Autodesk Inventor part; units mm, degrees
ref_plane "YZ Plane" through (0, 0, 0) normal (1, 0, 0) x (0, 1, 0)
ref_plane "XZ Plane" through (0, 0, 0) normal (0, 1, 0) x (-1, 0, 0)
ref_plane "XY Plane" through (0, 0, 0) normal (0, 0, 1) x (1, 0, 0)
sketch "Sketch1" plane through (0, 0, 0) normal (0, 1, 0) x (-1, 0, 0)
  line L0 (5, 5) -> (-5, 5)
  line L1 (-5, 5) -> (-5, -5)
  line L2 (-5, -5) -> (5, -5)
  line L3 (5, -5) -> (5, 5)
  line L4 (6, 6) -> (-6, 6)
  line L5 (-6, 6) -> (-6, -6)
  line L6 (-6, -6) -> (6, -6)
  line L7 (6, -6) -> (6, 6)
  point P0 (0, 0)
  dimension "d0" = 10
  dimension "d1" = 10
  dimension "d2" = 5
  dimension "d3" = 5
  dimension "d4" = 12
  dimension "d5" = 12
  dimension "d6" = 1
  dimension "d7" = 1
extrude "Extrusion1" add sketch "Sketch1" along normal blind 2
sketch "Sketch2" plane through (6, 0, 6) normal (1, 0, 0) x (0, 0, -1)
  line L0 (0, 0) -> (0, 2)
  line L1 (12, 0) -> (12, 2)
  line L2 (0, 2) -> (12, 2)
  line L3 (12, 2) -> (12, 1)
  line L4 (12, 1) -> (0, 1)
  line L5 (0, 1) -> (0, 2)
  point P0 (6, 0)
extrude "Extrusion2" add sketch "Sketch2" against normal blind 11.5
sketch "Sketch3" plane through (0, 2, 0) normal (0, 1, 0) x (1, 0, 0)
  line L0 (-2, -2) -> (2, -2)
  line L1 (2, -2) -> (2, 2)
  line L2 (2, 2) -> (-2, 2)
  line L3 (-2, 2) -> (-2, -2)
  circle A0 centre (0, 0) radius 2.8284
  line L4 (0, -2.8284) -> (-2.8284, 0)
  line L5 (-2.8284, 0) -> (0, 2.8284)
  line L6 (2.8284, 0) -> (0, 2.8284)
  line L7 (2.8284, 0) -> (0, -2.8284)
  point P0 (0.8284, -2)
  point P1 (2, -0.8284)
  point P2 (2, 0.8284)
  point P3 (0.8284, 2)
  point P4 (-0.8284, 2)
  point P5 (-2, 0.8284)
  point P6 (-2, -0.8284)
  point P7 (-0.8284, -2)
  dimension "d13" = 4
  dimension "d14" = 4
  dimension "d15" = 2
  dimension "d16" = 2
extrude "Extrusion3" cut sketch "Sketch3" along normal blind 23.25 and the other way blind 11.625 contours L4 L3 L5 L2 L6 L1 L7 L0
sketch "Sketch4" plane through (0, 2, 0) normal (0, 1, 0) x (1, 0, 0)
  line L0 (2, -0.8284) -> (2, 0.8284)
  line L1 (2, -0.8284) -> (2.8765, -0.8284)
  line L2 (2.8765, -0.8284) -> (2.8765, 0.8284)
  line L3 (2.8765, 0.8284) -> (2, 0.8284)
  line L4 (2, 0.8284) -> (2, -0.8284)
  line L5 (2.8765, -0.8284) -> (7.5124, -0.8284)
  line L6 (7.5124, -0.8284) -> (7.5124, 0.8284)
  line L7 (7.5124, 0.8284) -> (2.8765, 0.8284)
  line L8 (2.8765, 0.8284) -> (2.8765, -0.8284)
  point P0 (0, 0)
  point P1 (2.8765, 0.8284)
  point P2 (2, 0.8284)
extrude "Extrusion4" cut sketch "Sketch4" against normal blind 1
sketch "Sketch5" plane through (0, 2, 0) normal (0, 1, 0) x (1, 0, 0)
  line L0 (-6, -6) -> (6, -6)
  line L1 (6, 0.8284) -> (6, 6)
  line L2 (-6, -6) -> (6, -6)
  line L3 (6, -6) -> (6, 6)
  line L4 (6, 6) -> (-6, 6)
  line L5 (-6, 6) -> (-6, -6)
  point P0 (0, 0)
  point P1 (6, -6)
extrude "Extrusion5" add sketch "Sketch5" along normal blind 25
sketch "Sketch6" plane through (6, 0, 6) normal (1, 0, 0) x (0, 0, -1)
  line L0 (5.1716, 1) -> (5.1716, 2)
  line L1 (5.1716, 2) -> (-3.596, 2)
  line L2 (0, 0) -> (0, 27)
  line L3 (4, 2) -> (5.1716, 2)
  line L4 (5.1716, 2) -> (16.1787, 2)
  line L5 (5.1716, 2) -> (6.8284, 2)
  line L6 (6, 2) -> (6, 6)
  line L7 (0, 2) -> (6, 4)
  line L8 (6, 4) -> (12, 2)
  line L9 (12, 0) -> (12, 27)
  line L10 (12, 2) -> (-2.4689, 2)
  line L11 (-2.4689, 2) -> (-2.4689, 28.669)
  line L12 (-2.4689, 28.669) -> (12, 28.669)
  line L13 (12, 28.669) -> (12, 2)
  point P0 (6, 0)
  dimension "d23" = 4
extrude "Extrusion6" cut sketch "Sketch6" against normal blind 23.25 contours L1 L11 L12 L13 L9 L8 L7
sketch "Sketch7" plane through (-6, 0, 6) normal (0, 0, 1) x (1, 0, 0)
  line L0 (6, 0) -> (6, 4)
  line L1 (12, 4) -> (0, 4)
  line L2 (0, 2) -> (12, 2)
  line L3 (12, 2) -> (6, 4)
  line L4 (0, 4) -> (0, 2)
  line L5 (6, 4) -> (0, 2)
  line L6 (0, 2) -> (13.6732, 2)
  line L7 (13.6732, 2) -> (13.6732, 4.9606)
  line L8 (13.6732, 4.9606) -> (0, 4.9606)
  line L9 (0, 4.9606) -> (0, 2)
extrude "Extrusion7" cut sketch "Sketch7" against normal blind 41.75 contours L5 L4 L1 | L1 L9 L8 L7 L6 L3
sketch "Sketch8" plane through (0, 2, 0) normal (0, -1, 0) x (1, 0, 0)
  line L0 (6, 6) -> (0, 0)
  line L1 (1.9974, 1.9974) -> (-2.0026, 1.9974)
  line L2 (-2.0026, 1.9974) -> (-2.0026, -2.0026)
  line L3 (-2.0026, -2.0026) -> (1.9974, -2.0026)
  line L4 (1.9974, -2.0026) -> (1.9974, 1.9974)
  dimension "d30" = 4
  dimension "d31" = 4
extrude "Extrusion8" cut sketch "Sketch8" against normal blind 105
sketch "Sketch9" plane through (6, 0, 6) normal (1, 0, 0) x (0, 0, -1)
  line L0 (0, 0) -> (0, 2)
  line L1 (12, 0) -> (12, 2)
  line L2 (0, 0) -> (12, 0)
  line L3 (12, 0) -> (12, 2)
  line L4 (12, 2) -> (0, 2)
  line L5 (0, 2) -> (0, 0)
  point P0 (6, 0)
extrude "Extrusion9" add sketch "Sketch9" along normal blind 10
sketch "Sketch10" plane through (0, 0, 0) normal (0, -1, 0) x (1, 0, 0)
  line L0 (5, -5) -> (5, 5)
  line L1 (5, 5) -> (15, 5)
  line L2 (15, 5) -> (15, -5)
  line L3 (15, -5) -> (5, -5)
  line L4 (5, -5) -> (5, 5)
  point P0 (0, 0)
  dimension "d36" = 10
extrude "Extrusion10" cut sketch "Sketch10" against normal up to surface (1 mm away)
sketch "Sketch11" plane through (6, 2, 6) normal (0, 1, 0) x (1, 0, 0)
  line L0 (10, 0) -> (10, 12)
  line L1 (0, 0) -> (-4.0026, 4.0026)
  line L2 (10, 12) -> (-4.0026, 12)
  line L3 (-4.0026, 12) -> (-4.0026, 4.0026)
  line L4 (-4.0026, 4.0026) -> (10, 4.0026)
  line L5 (10, 4.0026) -> (10, 12)
  line L6 (-12, 0) -> (10, 0)
  line L7 (-4.0026, 4.0026) -> (10, 4.0026)
  line L8 (10, 4.0026) -> (10, 0)
  line L9 (10, 0) -> (-4.0026, 0)
  line L10 (-4.0026, 0) -> (-4.0026, 4.0026)
  point P0 (-6, 6)
extrude "Extrusion11" add sketch "Sketch11" along normal blind 1.5 contours L6 L1 L4 L0 | L4 L3 L2 L0
sketch "Sketch12" plane through (16, 0, 6) normal (1, 0, 0) x (0, 0, -1)
  line L0 (0, 2) -> (12, 2)
  line L1 (4.0026, 3.3342) -> (0, 2)
  line L2 (4.0026, 2) -> (4.0026, 3.3342)
  line L3 (0, 2) -> (4.0026, 3.3342)
  line L4 (4.0026, 3.3325) -> (8.0026, 3.3325)
  line L5 (4.0026, 3.3342) -> (8.0026, 3.3325)
  line L6 (12, 0) -> (12, 2)
  line L7 (8.0026, 3.3325) -> (12, 2)
  line L8 (0, 2) -> (-1.9464, 6.2775)
  line L9 (-1.9464, 6.2775) -> (14.9869, 5.8247)
  line L10 (14.9869, 5.8247) -> (12, 2)
  point P0 (6, 0)
extrude "Extrusion12" cut sketch "Sketch12" against normal blind 26 contours L8 L9 L10 L7 L4 L1
sketch "Sketch13" plane through (-6, 0, 6) normal (0, 0, 1) x (1, 0, 0)
  line L0 (3.9974, 2) -> (3.9974, 3.3325)
  line L1 (4.0026, 3.3342) -> (0, 2)
  line L2 (3.9974, 3.3325) -> (0, 3.3325)
  line L3 (0, 3.3325) -> (0, 2)
  line L4 (0, 2) -> (3.9974, 2)
  line L5 (3.9974, 2) -> (3.9974, 3.3325)
  line L6 (22, 2) -> (0, 2)
  line L7 (22, 3.3342) -> (4.0026, 3.3342)
  line L8 (22, 2) -> (18.0026, 2)
  line L9 (18.0026, 2) -> (18.0026, 3.3342)
  line L10 (18.0026, 3.3342) -> (22, 3.3342)
  line L11 (22, 3.3342) -> (22, 2)
  line L12 (18.0026, 3.3342) -> (22, 2)
  point P0 (6, 0)
  dimension "d43" = 3.9974
  dimension "d44" = 3.9974
extrude "Extrusion13" cut sketch "Sketch13" against normal blind 17.75 contours L12 L7 L11
sketch "Sketch14" plane through (-5, 1, -5) normal (0, -1, 0) x (1, 0, 0)
  line L0 (11, 5.8284) -> (11, 4.1716)
  line L1 (11, 5.8284) -> (19.699, 5.8284)
  line L2 (19.699, 5.8284) -> (19.699, 4.1716)
  line L3 (19.699, 4.1716) -> (11, 4.1716)
  line L4 (11, 4.1716) -> (11, 5.8284)
  line L5 (19.699, 4.1716) -> (21.7329, 4.1716)
  line L6 (21.7329, 4.1716) -> (21.7329, 5.8284)
  line L7 (21.7329, 5.8284) -> (19.699, 5.8284)
  line L8 (19.699, 5.8284) -> (19.699, 4.1716)
  point P0 (5, 5)
extrude "Extrusion14" cut sketch "Sketch14" against normal up to surface (1 mm away)
sketch "Sketch15" plane through (0, 0, 0) normal (0, -1, 0) x (1, 0, 0)
  point P0 (0, 0)
equation "\"d44\" = d43"
equation "\"BendRadius\" = Thickness"
equation "\"BendReliefWidth\" = Thickness"
equation "\"BendReliefDepth\" = 0.5 * Thickness"
equation "\"CornerReliefSize\" = 4 * Thickness"
equation "\"MinimumRemnant\" = 2 * Thickness"
equation "\"TransitionRadius\" = BendRadius"
equation "\"JacobiRadiusSize\" = BendRadius"
equation "\"GapSize\" = Thickness"
properties part number "modelGatePoklice1"
Can you work these out from the model? Positions are in its coordinate system, mm. A direction names the side the tool comes from. Round coordinates to 2 decimals unless told otherwise and drop trailing zeros. Loops run counter-clockwise (first coordinate to the right, second up) from the corner with the lowest first, then second, coordinate; pieces in that order, holes last. Notation, with made-up numbers: (-27, -11) - (12, -11) arc R29 ccw to (12, 21) - close; hole circle Ø1 at (-33.5, 61.25). An arc over 180 degrees is marked (long way). Write item = value, one per line. Start each with the question number.
(1) For P1, Ø0.8, axis at x = 15.5, z = 0, coming from the +Y side; P2, Ø1, axis at x = 7.5, z = 3, coming from the -Y side; P3, Ø1.5, axis at x = -3.5, z = -4, coming from the +Y side, each with a flat end and sliding along its axis, tell me the tip position at first contact or that it passes through.
(2) For faces 4 (the face through (-1.42, 1.49, -1.41)), 5 (the face through (15.5, 1, 0)), 6 (the face through (15, 0.5, 0.1)), 7 (the face through (-1.6, 2, -1.5)), which set-ups out of +Z, -Z, +X, -X, +Y, -Y let a thin tool reach every point of the face, with its end or its side?
(3) If we section it at B-B (x = -1.75): Please give me the cut outline in (y, z), and give its area (3 significant figures).
(4) If we mould it in two halves opening along X, with no side actions, what happens to faces 1 (the face through (16, 0.8, 0.1)), 2 (the face through (9.1, 1.5, -0.828)), 3 (the face through (0, 3, -2.003))? For each: released by +X, released by -X, zero draft, split by the parting line, or undercut.
(5) If I drill on probe 1 along Z at (x, y) = (0, 0.6); probe 2 along X at (y, z) = (0.7, -1.25); probe 3 along Z at (x, y) = (0.5, 1.8), over which ranges is the centre line in solid material (lowest first)? Write a range as [from, to].
(6) If we section it at D-D (x = 5): Please give me the cut outline in (y, z).
(7) If we section it at A-A (y = 0.3): Please give me the cut outline in (x, z).
Ans:
q1.P1 = 2.3
q1.P2 = 1
q1.P3 = 2.91
q2.face_4 = +Y, -Y
q2.face_5 = +X
q2.face_6 = -Y
q2.face_7 = +Y
q3.outline = (0, -6) - (2, -6) - (3.33, -2) - (2, -2) - (2, -1.08) - (1, -1.08) - (1, -5) - (0, -5) - close; (0, 5) - (1, 5) - (1, 1.08) - (2, 1.08) - (2, 2) - (3.33, 2) - (2, 6) - (0, 6) - close
q3.area = 17.2 mm²
q4.face_1 = released by +X
q4.face_2 = zero draft
q4.face_3 = undercut
q5.probe_1 = [-6, -5], [5, 6]
q5.probe_2 = [-6, -5], [15, 16]
q5.probe_3 = [-6, -2], [2, 6]
q6.outline = (0, -6) - (2, -6) - (3.33, -2) - (3.33, 2) - (2, 6) - (0, 6) - (0, 5) - (1, 5) - (1, 0.83) - (2, 0.83) - (2, -0.83) - (1, -0.83) - (1, -5) - (0, -5) - close
q7.outline = (-6, -6) - (16, -6) - (16, 6) - (-6, 6) - close; hole (-5, -5) - (15, -5) - (15, 5) - (-5, 5) - close
